```python
from build123d import *

# Parameters (mm, degrees)
SKETCH_1_R          = 12.5
EXTRUDE_1_DEPTH     = 5
SKETCH_2_R          = 4
EXTRUDE_2_DEPTH     = 2
SKETCH_3_R          = 3
EXTRUDE_3_DEPTH     = 13
SKETCH_4_R          = 1.65
CUT_EXTRUDE_1_DEPTH = 24.184046239


with BuildPart() as part:
    # ｽｹｯﾁ1 → ﾎﾞｽ - 押し出し1 (new body)
    with BuildSketch(Plane.XY):
        Circle(SKETCH_1_R)
    extrude(amount=EXTRUDE_1_DEPTH)

    # ｽｹｯﾁ2 → ﾎﾞｽ - 押し出し2 (add)
    with BuildSketch(Plane.XY.offset(5)):
        Circle(SKETCH_2_R)
    extrude(amount=EXTRUDE_2_DEPTH)

    # ｽｹｯﾁ3 → ﾎﾞｽ - 押し出し3 (add)
    with BuildSketch(Plane.XY.offset(7)):
        Circle(SKETCH_3_R)
    extrude(amount=EXTRUDE_3_DEPTH)

    # ｽｹｯﾁ4 → ｶｯﾄ - 押し出し1 (cut, through all)
    with BuildSketch(Plane.XY.offset(5)):
        with Locations((0, 7.5)):
            Circle(SKETCH_4_R)
        with Locations((7.5, 0)):
            Circle(SKETCH_4_R)
        with Locations((0, -7.5)):
            Circle(SKETCH_4_R)
        with Locations((-7.5, 0)):
            Circle(SKETCH_4_R)
    extrude(amount=-CUT_EXTRUDE_1_DEPTH, mode=Mode.SUBTRACT)


solid = part.part
```
Geometry check sheet. Reference: the model listing, model coordinates, mm. A direction names the side the tool comes from. Give positions to 0.01 mm unless a question says otherwise; leave off trailing zeros. Loops run counter-clockwise (first coordinate to the right, second up) from the corner with the lowest first, then second, coordinate; pieces in that order, holes last. Notation, with made-up numbers: (73.25, 13) - (122.25, 13) arc R16 ccw to (122.25, 34) - close; hole circle Ø6 at (-36, 46.5). An arc over 180 degrees is marked (long way). Use CSV: the item, a comma, the result in double quotes. Start each with the question number.
Q1. Section check B-B, the plane y = 0. Record the cut outline in (x, z).
Q2. Scan lines: probe 1 along Y at (x, z) = (0, 1.55); probe 2 along Z at (x, y) = (8.25, 7.5); probe 3 along Y at (x, z) = (-7.5, 1.1). Record each from-to range of solid material in increasing order. Write a range as from..to.
Q3. Go/stop test with flat-tipped pins: pin 1 Ø8 at (x, z) = (3.5, 13) entering from +Y; pin 2 Ø2 at (y, z) = (5.5, 5.5) entering from -X; pin 3 Ø4.5 at (x, y) = (7.5, 0) entering from +Z. Record where each tip stops, or that it passes through.
Q4. Access from +Z, -Z, +X, -X, +Y, -Y to the whole of each face (thin tool, end or side, straight path). Record for faces 5 (the face through (-3, 3, 5)), 6 (the face through (-1.216, 8.615, 2.535)).
Q5. Section check A-A, the plane x = -7.5. Record the cut outline in (y, z).
Q6. Release check for a two-part mould opening along X. For faces 1 (the face through (5.85, 0.07, 2.54)), 2 (the face through (11.923, 3.755, 2.465)), 3 (the face through (0, 0, 0)), 4 (the face through (-9.15, 0.07, 2.54)) record: +X half, -X half, draft (parallel to the pull), parting line (faces both ways), or undercut.
Findings below:
1,outline,"(-12.5, 0) - (-9.15, 0) - (-9.15, 5) - (-12.5, 5) - close; (-5.85, 0) - (5.85, 0) - (5.85, 5) - (4, 5) - (4, 7) - (3, 7) - (3, 20) - (-3, 20) - (-3, 7) - (-4, 7) - (-4, 5) - (-5.85, 5) - close; (9.15, 0) - (12.5, 0) - (12.5, 5) - (9.15, 5) - close"
2,probe 1,"y = -12.5..-9.15, -5.85..5.85, 9.15..12.5"
2,probe 2,"z = 0..5"
2,probe 3,"y = -10..-1.65, 1.65..10"
3,pin 1,"stops at y = 3"
3,pin 2,"stops at x = -11.61"
3,pin 3,"stops at z = 5"
4,face 5,"+Z"
4,face 6,"+Z, -Z"
5,outline,"(-10, 0) - (-1.65, 0) - (-1.65, 5) - (-10, 5) - close; (1.65, 0) - (10, 0) - (10, 5) - (1.65, 5) - close"
6,face 1,"undercut"
6,face 2,"parting line"
6,face 3,"draft"
6,face 4,"undercut"
